Design review of the part built by this model. Coordinates are the model's own, in mm. Coordinates: 2 decimals unless noted, no trailing zeros. Order: outer loops, then holes, each group sorted by start corner. A loop starts at its lowest first (then second) coordinate and runs counter-clockwise, first axis right, second up. Notation, with made-up numbers: (2, 53.5) -> (14, 53.5) arc R33 ccw to (14, 86.5) -> close; hole circle Ø9 at (14.5, 61). An arc over 180 degrees is marked (long way). Write item = value, one per line.
```python
from build123d import *

# Parameters (mm, degrees)
SKETCH_1_R          = 1.5
EXTRUDE_1_DEPTH     = 2
FILLET_1_R          = 2
SKETCH_2_W          = 1
SKETCH_2_H          = 1
CUT_EXTRUDE_1_DEPTH = 50


with BuildPart() as part:
    # 草图1 → 凸台-拉伸1 (new body)
    with BuildSketch(Plane.XY):
        with BuildLine():
            Line((0, 6.560739839), (10, 6.560739839))
            ThreePointArc((10, 6.560739839), (16.560739839, 0), (10, -6.560739839))
            Line((10, -6.560739839), (0, -6.560739839))
            ThreePointArc((0, -6.560739839), (-6.560739839, 0), (0, 6.560739839))
        make_face()
        Circle(SKETCH_1_R, mode=Mode.SUBTRACT)
        with Locations((10, 0)):
            Circle(SKETCH_1_R, mode=Mode.SUBTRACT)
    extrude(amount=EXTRUDE_1_DEPTH)

    # 圆角1
    fillet_1_edges = [part.edges().sort_by_distance(p)[0] for p in [
        (8.5, 0, 2),
        (5, 6.560739839, 2),
        (16.560739839, 0, 2),
        (5, -6.560739839, 2),
        (-6.560739839, 0, 2),
        (-1.5, 0, 2),
    ]]
    fillet(fillet_1_edges, radius=FILLET_1_R - 0.0001)  # a hair under: the kernel refuses the full size

    # 草图2 → 切除-拉伸1 (cut, symmetric)
    with BuildSketch(Plane(origin=(0, 0, 0), x_dir=(1, 0, 0), z_dir=(0, 1, 0))):
        with Locations((5, -2)):
            Rectangle(SKETCH_2_W, SKETCH_2_H)
    extrude(amount=CUT_EXTRUDE_1_DEPTH, both=True, mode=Mode.SUBTRACT)


solid = part.part
```
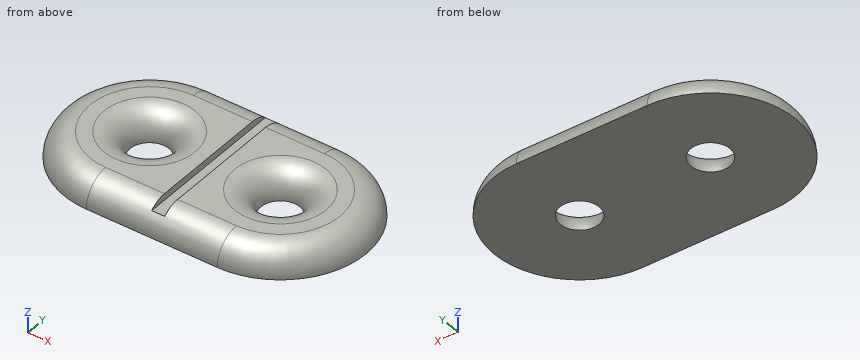
(1) We need section B-B (z = 1.05). Write out the cut boundary in (x, y).
Report:
outline = (0, -6.26) -> (10, -6.26) arc R6.26 ccw to (10, 6.26) -> (0, 6.26) arc R6.26 ccw to start; hole circle Ø3.6 at (0, 0); hole circle Ø3.6 at (10, 0)
(2) Insertion check: pin 1 (0.5 mm diameter, centred on x = 5, y = 1.5, fed in from +Z); pin 2 (4 mm diameter, centred on x = 0, y = 0, fed in from -Z); pin 3 (1 mm diameter, centred on x = 2, z = 1.5, fed in from -Y). Each pin has a flat end and moves straight along its axis. Give the tip position at first contact, or say it passes through.
Report:
pin_1 = 1.5
pin_2 = 0
pin_3 = -6.29
(3) We need section A-A (y = 0). Give the number of separate pieces and of enclosed holes in the cut face, and give its area (3 significant figures).
Report:
separate_pieces = 3
enclosed_holes = 0
area = 28.6 mm²
(4) For L1, parallel to Y at x = 10, z = 0.05; L2, parallel to Z at x = 5.25, y = -3.5; L3, parallel to X at y = -2.5, z = 1.7, list the stretches that pass through material, from the lowest coordinate up.
Report:
L1 = -6.56 to -1.5, 1.5 to 6.56
L2 = 0 to 1.5
L3 = -5.03 to 4.5, 5.5 to 15.03
